Geometry: final body of the model. Coordinates: model frame, mm. Coordinates: 2 decimals unless noted, no trailing zeros. Loops run counter-clockwise (first coordinate to the right, second up) from the corner with the lowest first, then second, coordinate; pieces in that order, holes last. Notation, with made-up numbers: (59, 66) - (101, 66) arc R34 cw to (101, 104) - close; hole circle Ø11 at (-18.75, 68.25). An arc over 180 degrees is marked (long way). Put each result on its own line as item: value. Start each with the question number.
1) Section C-C on y = -7.5. Output: boundary loops of the cut face in (x, z).
2) Section D-D on y = 3.5. Output: boundary loops of the cut face in (x, z), and give its area (3 significant figures).
3) Material intervals for line 1 along Y through (x, z) = (25, 0.8); line 2 along Y through (x, z) = (32.5, 0.95); line 3 along X through (y, z) = (-1.25, 0.7), sorted ascending. Write a range as from..to.
4) Section A-A on y = 0. Output: boundary loops of the cut face in (x, z).
5) Section B-B on z = 0.65. Output: boundary loops of the cut face in (x, y), and give its area (3 significant figures).
6) Contact query for a flat-ended pin moving along its axis: pin 1 Ø3 at (x, y) = (32.59, -7.5) entering from -Z. Output: stop coordinate, or through.
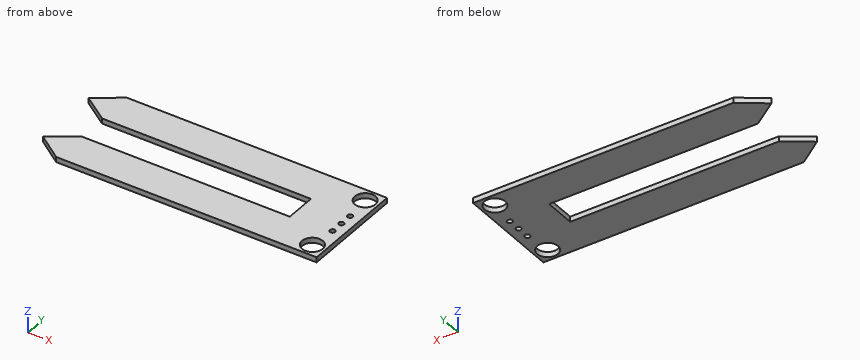
```python
from build123d import *

# Parameters (mm, degrees)
SKETCH_R   = 2
SKETCH_R_2 = 0.5
PAD_DEPTH  = 1


with BuildPart() as part:
    # Sketch → Pad (new body)
    with BuildSketch(Plane.XY):
        Polygon((35.093211, 10), (35.093211, -10), (-14.906789, -10), (-19.819749, -6.468102), (-14.861446, -3.000147), (25.216118, -3.000147), (25.216118, 3.000147), (-14.861446, 3.000147), (-19.819749, 6.468102), (-14.906789, 10), align=None)
        with Locations((32.593211, 7.5)):
            Circle(SKETCH_R, mode=Mode.SUBTRACT)
        with Locations((32.593211, -7.5)):
            Circle(SKETCH_R, mode=Mode.SUBTRACT)
        with Locations((33.093211, 2.5)):
            Circle(SKETCH_R_2, mode=Mode.SUBTRACT)
        with Locations((33.093211, 0)):
            Circle(SKETCH_R_2, mode=Mode.SUBTRACT)
        with Locations((33.093211, -2.5)):
            Circle(SKETCH_R_2, mode=Mode.SUBTRACT)
    extrude(amount=PAD_DEPTH)


solid = part.part
```
Answer block:
1. outline: (-18.38, 0) - (30.59, 0) - (30.59, 1) - (-18.38, 1) - close; (34.59, 0) - (35.09, 0) - (35.09, 1) - (34.59, 1) - close
2. outline: (-15.58, 0) - (35.09, 0) - (35.09, 1) - (-15.58, 1) - close
2. area: 50.7 mm²
3. line 1: y = -10..-3, 3..10
3. line 2: y = -10..-9.5, -5.5..5.5, 9.5..10
3. line 3: x = 25.22..35.09
4. outline: (25.22, 0) - (32.59, 0) - (32.59, 1) - (25.22, 1) - close; (33.59, 0) - (35.09, 0) - (35.09, 1) - (33.59, 1) - close
5. outline: (-19.82, -6.47) - (-14.91, -10) - (35.09, -10) - (35.09, 10) - (-14.91, 10) - (-19.82, 6.47) - (-14.86, 3) - (25.22, 3) - (25.22, -3) - (-14.86, -3) - close; hole circle Ø4 at (32.59, -7.5); hole circle Ø4 at (32.59, 7.5); hole circle Ø1 at (33.09, -2.5); hole circle Ø1 at (33.09, 0); hole circle Ø1 at (33.09, 2.5)
5. area: 766 mm²
6. pin 1: passes through
